from build123d import *

# Parameters (mm, degrees)
SKETCH_W        = 31.75
SKETCH_H        = 31.75
PAD_DEPTH       = 63.5
SKETCH001_R     = 11
POCKET_DEPTH    = 7
SKETCH002_R     = 8
POCKET001_DEPTH = 31.751
SKETCH003_R     = 1.25
HOLE_DEPTH      = 31.751
SKETCH004_R     = 4.25
HOLE001_DEPTH   = 25


with BuildPart() as part:
    # Sketch → Pad (new body)
    with BuildSketch(Plane.XY):
        Rectangle(SKETCH_W, SKETCH_H)
    extrude(amount=PAD_DEPTH)

    # Sketch001 (on Face2 of Pad) → Pocket (cut)
    with BuildSketch(Plane.XZ.offset(15.875)):
        with Locations((0, 19.05)):
            Circle(SKETCH001_R)
    pocket = extrude(amount=-POCKET_DEPTH, mode=Mode.SUBTRACT)

    # Mirrored: Pocket across XZ
    add(pocket.mirror(Plane.XZ), mode=Mode.SUBTRACT)

    # Sketch002 (on Face3 of Mirrored) → Pocket001 (cut, through all)
    with BuildSketch(Plane.XZ.offset(15.875)):
        with Locations((0, 19.05)):
            Circle(SKETCH002_R)
    extrude(amount=-POCKET001_DEPTH, mode=Mode.SUBTRACT)

    # Sketch003 (on Face1 of Pocket001) → Hole (cut, through all)
    with BuildSketch(Plane(origin=(-15.875, 0, 0), x_dir=(0, -1, 0), z_dir=(-1, 0, 0))):
        with Locations((12.5, 31.55)):
            Circle(SKETCH003_R)
        with Locations((12.5, 6.55)):
            Circle(SKETCH003_R)
        with Locations((-12.5, 6.55)):
            Circle(SKETCH003_R)
        with Locations((-12.5, 31.55)):
            Circle(SKETCH003_R)
    extrude(amount=-HOLE_DEPTH, mode=Mode.SUBTRACT)

    # Sketch004 (on Face4 of Hole) → Hole001 (cut)
    with BuildSketch(Plane.XY.offset(63.5)):
        Circle(SKETCH004_R)
    extrude(amount=-HOLE001_DEPTH, mode=Mode.SUBTRACT)


solid = part.part
Model file for the job. Use its own axes, mm. A direction names the side the tool comes from. Coordinates: 2 decimals unless noted, no trailing zeros. Loops run counter-clockwise (first coordinate to the right, second up) from the corner with the lowest first, then second, coordinate; pieces in that order, holes last. Notation, with made-up numbers: (38, 15.5) -> (59, 15.5) arc R3 cw to (59, 19.5) -> close; hole circle Ø7 at (66, 52.5). An arc over 180 degrees is marked (long way). Use one line per item in the form item = value. Start each with the question number.
(1) Pull direction Z, two halves, no side cores. Call faces 1 (the flat face through (0, 0, 0)), 2 (the flat face through (3, 4, 63.5)), 3 (the flat face through (0, -15.875, 31)), 4 (the cylindrical face through (-2.38, -12.42, 8.31)): pulls with the +Z half, pulls with the -Z half, needs draft (parallel to the pull), parting line crosses it, or undercut.
(2) Cut at A-A on y = -12.5. Give the cut face in (x, z) (3 decimals), and give its area (3 significant figures).
(3) Cut at C-C on z = 31.55. Give the cut face in (x, y) (3 decimals).
(4) Probe probe 1 along Z at (x, y) = (0, -12.5); probe 2 along Z at (x, y) = (-6.5, -12); probe 3 along X at (y, z) = (13, 19) (3 decimals). List the from-to ranges inside material, lowest first. Write a range as from..to.
(5) Flat gauge pins, fed straight in: pin 1 (2 mm diameter, centred on y = -12.5, z = 31.55, fed in from -X); pin 2 (5 mm diameter, centred on x = -12, y = -6.5, fed in from -Z); pin 3 (1 mm diameter, centred on x = 3, z = 10.5, fed in from +Y) (3 decimals). Where does each tip first touch, or does it go through?
(6) Cut at B-B on x = 0. Give the cut face in (y, z) (3 decimals).
(7) Cut at D-D on z = 46.5. Give the cut face in (x, y) (3 decimals), and give its area (3 significant figures).
(8) Tool access for faces 5 (the flat face through (-2, -8.875, 11)), 6 (the flat face through (0, 0, 38.5)), 7 (the flat face through (-2, 8.875, 11)), 8 (the cylindrical face through (7.63, -0.12, 21.45)): list every direction of +Z, -Z, +X, -X, +Y, -Y with a clear straight run to the whole face (end or side of a thin tool).
Values:
q1.face_1 = pulls with the -Z half
q1.face_2 = pulls with the +Z half
q1.face_3 = needs draft
q1.face_4 = undercut
q2.outline = (-15.875, 0) -> (15.875, 0) -> (15.875, 5.3) -> (-15.875, 5.3) -> close; (-15.875, 7.8) -> (15.875, 7.8) -> (15.875, 30.3) -> (-15.875, 30.3) -> close; (-15.875, 32.8) -> (15.875, 32.8) -> (15.875, 63.5) -> (-15.875, 63.5) -> close; hole circle Ø22 at (0, 19.05)
q2.area = 1,480 mm2
q3.outline = (-15.875, -15.875) -> (15.875, -15.875) -> (15.875, -13.75) -> (-15.875, -13.75) -> close; (-15.875, -11.25) -> (15.875, -11.25) -> (15.875, 11.25) -> (-15.875, 11.25) -> close; (-15.875, 13.75) -> (15.875, 13.75) -> (15.875, 15.875) -> (-15.875, 15.875) -> close
q4.probe_1 = 0..5.3, 7.8..8.05, 30.05..30.3, 32.8..63.5
q4.probe_2 = 0..5.4, 7.7..10.18, 27.92..30.4, 32.7..63.5
q4.probe_3 = -15.875..-11, 11..15.875
q5.pin_1 = through
q5.pin_2 = 0
q5.pin_3 = 8.875
q6.outline = (-15.875, 0) -> (15.875, 0) -> (15.875, 8.05) -> (8.875, 8.05) -> (8.875, 11.05) -> (-8.875, 11.05) -> (-8.875, 8.05) -> (-15.875, 8.05) -> close; (-15.875, 30.05) -> (-8.875, 30.05) -> (-8.875, 27.05) -> (8.875, 27.05) -> (8.875, 30.05) -> (15.875, 30.05) -> (15.875, 63.5) -> (4.25, 63.5) -> (4.25, 38.5) -> (-4.25, 38.5) -> (-4.25, 63.5) -> (-15.875, 63.5) -> close; hole circle Ø2.5 at (-12.5, 6.55); hole circle Ø2.5 at (-12.5, 31.55); hole circle Ø2.5 at (12.5, 6.55); hole circle Ø2.5 at (12.5, 31.55)
q7.outline = (-15.875, -15.875) -> (15.875, -15.875) -> (15.875, 15.875) -> (-15.875, 15.875) -> close; hole circle Ø8.5 at (0, 0)
q7.area = 951 mm2
q8.face_5 = -Y
q8.face_6 = +Z
q8.face_7 = +Y
q8.face_8 = +Y, -Y
